Input: dimensioned drawing with shaded views. Units: mm. Origin: part minimum x, y, z. Round coordinates to 2 decimals unless told otherwise and drop trailing zeros. Loops run counter-clockwise (first coordinate to the right, second up) from the corner with the lowest first, then second, coordinate; pieces in that order, holes last.
Item 1: Section query C-C on z = 6.5. Return loops of the section in (x, y), then the cut area to 3 significant figures.
Item 2: First-contact query: P1, Ø3.5, axis at x = 83.5, y = 8, coming from the +Z side; P2, Ø3, axis at x = 200.5, z = 5, coming from the -Y side; P3, Ø2, axis at x = 187, z = 5.5, coming from the +Y side. Flat tips, straight axial feed; report the tip coordinate or a pass-through.
Item 3: Section query B-B on x = 171.5. Return loops of the section in (y, z).
Item 4: Ray query, L1, parallel to Y at x = 12.5, z = 1.55; L2, parallel to Y at x = 64.5, z = 8. Return the intervals inside material, ascending.
Item 5: Section query A-A on y = 6.5. Return loops of the section in (x, z), then the cut area to 3 significant figures.
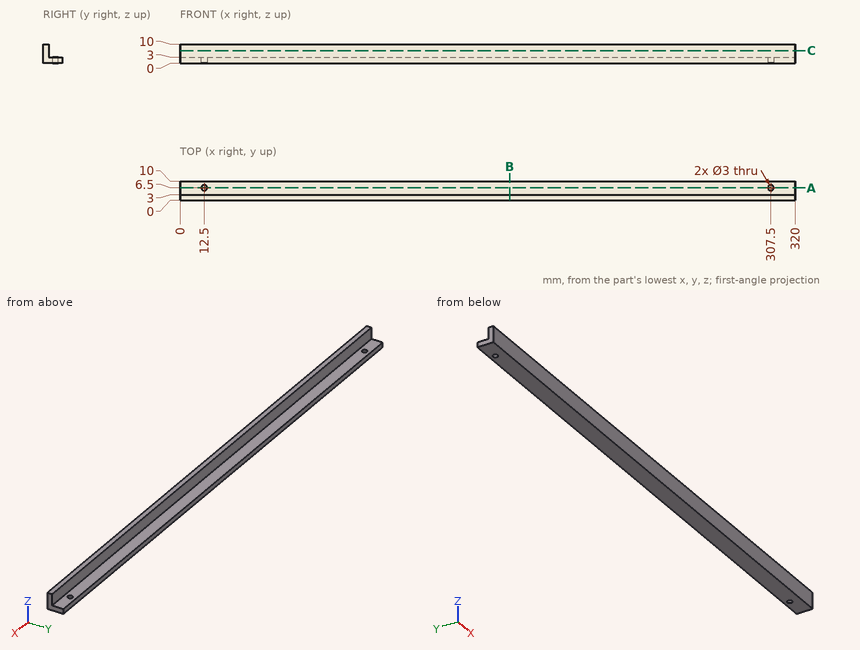
Data:
1. outline: (0, 0) - (320, 0) - (320, 3) - (0, 3) - close
1. area: 960 mm2
2. P1: stops at z = 3
2. P2: stops at y = 0
2. P3: stops at y = 3
3. outline: (0, 0) - (10, 0) - (10, 3) - (3, 3) - (3, 10) - (0, 10) - close
4. L1: y = 0 to 5, 8 to 10
4. L2: y = 0 to 3
5. outline: (0, 0) - (11, 0) - (11, 3) - (0, 3) - close; (14, 0) - (306, 0) - (306, 3) - (14, 3) - close; (309, 0) - (320, 0) - (320, 3) - (309, 3) - close
5. area: 942 mm2
